For this review, take the finished solid that the model builds, in its own axes (mm). A direction names the side the tool comes from. Give positions to 0.01 mm unless a question says otherwise; leave off trailing zeros. Write each loop counter-clockwise with the first axis right and the second up, starting at its lowest first coordinate (ties: lowest second). Pieces come first, ordered by that corner, then holes. Notation, with made-up numbers: (31.25, 12.25) -> (45.25, 12.25) arc R21 ccw to (45.25, 39.25) -> close; hole circle Ø2 at (13, 46). An arc over 180 degrees is marked (long way). Write item = value, one per line.
```python
from build123d import *

# Parameters (mm, degrees)
SKETCH1_W                    = 320
SKETCH1_H                    = 90.51
CHASSIS_BASE_DEPTH           = 5
SKETCH3_W                    = 2
SKETCH3_H                    = 275
LATERAL_GUARD_DEPTH          = 3
DRIVE_ATTACHMENT_POINT_REACH = 10
SKETCH4_R                    = 3
CUT_EXTRUDE2_REACH           = 7
SKETCH5_R                    = 6.5
SKETCH5_R_2                  = 1
SKETCH6_W                    = 30
SKETCH6_H                    = 30
BOSS_EXTRUDE1_DEPTH          = 90.51
CUT_EXTRUDE3_REACH           = 32
SKETCH7_W                    = 60
SKETCH7_H                    = 30
FILLET3_R                    = 0.5
FILLET4_R                    = 2
SKETCH9_R                    = 0.875
CUT_EXTRUDE5_DEPTH           = 5
SKETCH10_R                   = 0.875
CUT_EXTRUDE6_DEPTH           = 5
SKETCH11_R                   = 0.875
CUT_EXTRUDE7_DEPTH           = 5
SKETCH12_R                   = 0.875
CUT_EXTRUDE8_DEPTH           = 5
SKETCH13_R                   = 0.875
CUT_EXTRUDE9_DEPTH           = 5
SKETCH14_R                   = 0.875
CUT_EXTRUDE10_DEPTH          = 5
BOSS_EXTRUDE2_DEPTH          = 1.6
SKETCH17_R                   = 10.925
CUT_EXTRUDE12_DEPTH          = 91.51
SKETCH18_W                   = 18
SKETCH18_H                   = 15
CUT_EXTRUDE13_DEPTH          = 6.0000001
SKETCH23_R                   = 1.5
CUT_EXTRUDE18_DEPTH          = 35


with BuildPart() as part:
    # Sketch1 → Chassis Base (new body)
    with BuildSketch(Plane(origin=(0, 0, 0), x_dir=(0, 1, 0), z_dir=(0, 0, 1))):
        Rectangle(SKETCH1_W, SKETCH1_H)
    extrude(amount=CHASSIS_BASE_DEPTH)

    # Sketch3 → Lateral Guard (add)
    with BuildSketch(Plane.XY.offset(5)):
        with Locations((-44.255, 7.5)):
            Rectangle(SKETCH3_W, SKETCH3_H)
        with Locations((44.255, 7.5)):
            Rectangle(SKETCH3_W, SKETCH3_H)
    extrude(amount=LATERAL_GUARD_DEPTH)

    # Sketch4 → Drive Attachment Point (cut, up to next)
    with BuildSketch(Plane(origin=(0, 0, 0), x_dir=(1, 0, 0), z_dir=(0, 0, -1)), mode=Mode.PRIVATE) as drive_attachment_point_sk1:
        with Locations((0, -29.7)):
            Circle(SKETCH4_R)
    drive_attachment_point_tool1 = extrude(drive_attachment_point_sk1.sketch, amount=-DRIVE_ATTACHMENT_POINT_REACH, mode=Mode.PRIVATE) & part.part
    add(drive_attachment_point_tool1.solids().sort_by_distance((0, 29.7, 0))[0], mode=Mode.SUBTRACT)
    # Sketch4 → Drive Attachment Point (cut, up to next)
    with BuildSketch(Plane(origin=(0, 0, 0), x_dir=(1, 0, 0), z_dir=(0, 0, -1)), mode=Mode.PRIVATE) as drive_attachment_point_sk2:
        with Locations((-20.08, 30)):
            Circle(SKETCH4_R)
    drive_attachment_point_tool2 = extrude(drive_attachment_point_sk2.sketch, amount=-DRIVE_ATTACHMENT_POINT_REACH, mode=Mode.PRIVATE) & part.part
    add(drive_attachment_point_tool2.solids().sort_by_distance((-20.08, -30, 0))[0], mode=Mode.SUBTRACT)
    # Sketch4 → Drive Attachment Point (cut, up to next)
    with BuildSketch(Plane(origin=(0, 0, 0), x_dir=(1, 0, 0), z_dir=(0, 0, -1)), mode=Mode.PRIVATE) as drive_attachment_point_sk3:
        with Locations((20.08, 30)):
            Circle(SKETCH4_R)
    drive_attachment_point_tool3 = extrude(drive_attachment_point_sk3.sketch, amount=-DRIVE_ATTACHMENT_POINT_REACH, mode=Mode.PRIVATE) & part.part
    add(drive_attachment_point_tool3.solids().sort_by_distance((20.08, -30, 0))[0], mode=Mode.SUBTRACT)
    # Sketch4 → Drive Attachment Point (cut, up to next)
    with BuildSketch(Plane(origin=(0, 0, 0), x_dir=(1, 0, 0), z_dir=(0, 0, -1)), mode=Mode.PRIVATE) as drive_attachment_point_sk4:
        with Locations((0, 49.3)):
            Circle(SKETCH4_R)
    drive_attachment_point_tool4 = extrude(drive_attachment_point_sk4.sketch, amount=-DRIVE_ATTACHMENT_POINT_REACH, mode=Mode.PRIVATE) & part.part
    add(drive_attachment_point_tool4.solids().sort_by_distance((0, -49.3, 0))[0], mode=Mode.SUBTRACT)
    # Sketch4 → Drive Attachment Point (cut, up to next)
    with BuildSketch(Plane(origin=(0, 0, 0), x_dir=(1, 0, 0), z_dir=(0, 0, -1)), mode=Mode.PRIVATE) as drive_attachment_point_sk5:
        with Locations((-20.08, -10.4)):
            Circle(SKETCH4_R)
    drive_attachment_point_tool5 = extrude(drive_attachment_point_sk5.sketch, amount=-DRIVE_ATTACHMENT_POINT_REACH, mode=Mode.PRIVATE) & part.part
    add(drive_attachment_point_tool5.solids().sort_by_distance((-20.08, 10.4, 0))[0], mode=Mode.SUBTRACT)
    # Sketch4 → Drive Attachment Point (cut, up to next)
    with BuildSketch(Plane(origin=(0, 0, 0), x_dir=(1, 0, 0), z_dir=(0, 0, -1)), mode=Mode.PRIVATE) as drive_attachment_point_sk6:
        with Locations((20.08, -10.4)):
            Circle(SKETCH4_R)
    drive_attachment_point_tool6 = extrude(drive_attachment_point_sk6.sketch, amount=-DRIVE_ATTACHMENT_POINT_REACH, mode=Mode.PRIVATE) & part.part
    add(drive_attachment_point_tool6.solids().sort_by_distance((20.08, 10.4, 0))[0], mode=Mode.SUBTRACT)

    # Sketch5 → Cut-Extrude2 (cut, up to next)
    with BuildSketch(Plane.XY.offset(5), mode=Mode.PRIVATE) as cut_extrude2_sk1:
        with Locations((0, 148)):
            Circle(SKETCH5_R)
    cut_extrude2_tool1 = extrude(cut_extrude2_sk1.sketch, amount=-CUT_EXTRUDE2_REACH, mode=Mode.PRIVATE) & part.part
    add(cut_extrude2_tool1.solids().sort_by_distance((0, 148, 5))[0], mode=Mode.SUBTRACT)
    # Sketch5 → Cut-Extrude2 (cut, up to next)
    with BuildSketch(Plane.XY.offset(5), mode=Mode.PRIVATE) as cut_extrude2_sk2:
        with Locations((-17.5, 140.5)):
            Circle(SKETCH5_R_2)
    cut_extrude2_tool2 = extrude(cut_extrude2_sk2.sketch, amount=-CUT_EXTRUDE2_REACH, mode=Mode.PRIVATE) & part.part
    add(cut_extrude2_tool2.solids().sort_by_distance((-17.5, 140.5, 5))[0], mode=Mode.SUBTRACT)
    # Sketch5 → Cut-Extrude2 (cut, up to next)
    with BuildSketch(Plane.XY.offset(5), mode=Mode.PRIVATE) as cut_extrude2_sk3:
        with Locations((17.5, 140.5)):
            Circle(SKETCH5_R_2)
    cut_extrude2_tool3 = extrude(cut_extrude2_sk3.sketch, amount=-CUT_EXTRUDE2_REACH, mode=Mode.PRIVATE) & part.part
    add(cut_extrude2_tool3.solids().sort_by_distance((17.5, 140.5, 5))[0], mode=Mode.SUBTRACT)

    # Sketch6 → Boss-Extrude1 (add)
    with BuildSketch(Plane.YZ.offset(45.255)):
        with Locations((-145, 15)):
            Rectangle(SKETCH6_W, SKETCH6_H)
    extrude(amount=-BOSS_EXTRUDE1_DEPTH)

    # Sketch7 → Cut-Extrude3 (cut, up to next)
    with BuildSketch(Plane.XY.offset(30), mode=Mode.PRIVATE) as cut_extrude3_sk1:
        with Locations((0, -145)):
            Rectangle(SKETCH7_W, SKETCH7_H)
    cut_extrude3_tool1 = extrude(cut_extrude3_sk1.sketch, amount=-CUT_EXTRUDE3_REACH, mode=Mode.PRIVATE) & part.part
    add(cut_extrude3_tool1.solids().sort_by_distance((0, -145, 30))[0], mode=Mode.SUBTRACT)

    # Fillet3
    fillet3_edges = [part.edges().sort_by_distance(p)[0] for p in [
        (-45.255, 7.5, 8),
        (-43.255, 7.5, 8),
        (45.255, 7.5, 8),
        (43.255, 7.5, 8),
    ]]
    fillet(fillet3_edges, radius=FILLET3_R)

    # Fillet4
    fillet4_edges = [part.edges().sort_by_distance(p)[0] for p in [
        (37.6275, -130, 30),
        (-37.6275, -130, 30),
    ]]
    fillet(fillet4_edges, radius=FILLET4_R)

    # Sketch9 → Cut-Extrude5 (cut)
    with BuildSketch(Plane.XY.offset(30)):
        with Locations((-37.6275, -146)):
            Circle(SKETCH9_R)
    extrude(amount=-CUT_EXTRUDE5_DEPTH, mode=Mode.SUBTRACT)

    # Sketch10 → Cut-Extrude6 (cut)
    with BuildSketch(Plane.XZ.offset(160)):
        with Locations((-37.6275, 15)):
            Circle(SKETCH10_R)
    extrude(amount=-CUT_EXTRUDE6_DEPTH, mode=Mode.SUBTRACT)

    # Sketch11 → Cut-Extrude7 (cut)
    with BuildSketch(Plane(origin=(0, 0, 0), x_dir=(1, 0, 0), z_dir=(0, 0, -1))):
        with Locations((-37.6275, 148.599605515)):
            Circle(SKETCH11_R)
    extrude(amount=-CUT_EXTRUDE7_DEPTH, mode=Mode.SUBTRACT)

    # Sketch12 → Cut-Extrude8 (cut)
    with BuildSketch(Plane(origin=(0, 0, 0), x_dir=(1, 0, 0), z_dir=(0, 0, -1))):
        with Locations((37.6275, 145)):
            Circle(SKETCH12_R)
    extrude(amount=-CUT_EXTRUDE8_DEPTH, mode=Mode.SUBTRACT)

    # Sketch13 → Cut-Extrude9 (cut)
    with BuildSketch(Plane.XZ.offset(160)):
        with Locations((37.6275, 15)):
            Circle(SKETCH13_R)
    extrude(amount=-CUT_EXTRUDE9_DEPTH, mode=Mode.SUBTRACT)

    # Sketch14 → Cut-Extrude10 (cut)
    with BuildSketch(Plane.XY.offset(30)):
        with Locations((37.6275, -146)):
            Circle(SKETCH14_R)
    extrude(amount=-CUT_EXTRUDE10_DEPTH, mode=Mode.SUBTRACT)

    # Sketch15 → Boss-Extrude2 (add)
    with BuildSketch(Plane.XY.offset(5)):
        with BuildLine():
            Line((-17.021586315, 136.436061109), (17.021586315, 136.436061109))
            ThreePointArc((17.021586315, 136.436061109), (0, 123), (-17.021586315, 136.436061109))
        make_face()
    extrude(amount=BOSS_EXTRUDE2_DEPTH)

    # Sketch17 → Cut-Extrude12 (cut, through all)
    with BuildSketch(Plane(origin=(-45.255, 0, 0), x_dir=(0, -1, 0), z_dir=(-1, 0, 0))):
        with Locations((145, 15)):
            Circle(SKETCH17_R)
    extrude(amount=-CUT_EXTRUDE12_DEPTH, mode=Mode.SUBTRACT)

    # Sketch18 → Cut-Extrude13 (cut, through all)
    with BuildSketch(Plane.XY.offset(5)):
        with Locations((21, -122.5)):
            Rectangle(SKETCH18_W, SKETCH18_H)
        with Locations((-21, -122.5)):
            Rectangle(SKETCH18_W, SKETCH18_H)
    extrude(amount=-CUT_EXTRUDE13_DEPTH, mode=Mode.SUBTRACT)

    # Sketch21 → Revolve1 (revolve)
    with BuildSketch(Plane.YZ):
        with BuildLine():
            Line((-118, 40), (-118, 5))
            Line((-118, 5), (-106.234133627, 4.682586024))
            add(Edge.make_bspline(
                [(-115, 40), (-114.798550354, 20.795762888), (-106.234133627, 4.682586024)],
                knots=[0, 0, 0, 1, 1, 1], degree=2))
            Line((-115, 40), (-118, 40))
        make_face()
    revolve(axis=Axis((0, -118, 40), (0, 0, -1)))

    # Sketch23 → Cut-Extrude18 (cut)
    with BuildSketch(Plane(origin=(0, 0, 40), x_dir=(0, 1, 0), z_dir=(0, 0, 1))):
        with Locations((-118, 0)):
            Circle(SKETCH23_R)
    extrude(amount=-CUT_EXTRUDE18_DEPTH, mode=Mode.SUBTRACT)


solid = part.part
```
(1) Tool access review of faces 1 (the face through (30, -138, 5)), 2 (the face through (17.083, -30.132, 2.465)), 3 (the face through (0, 123, 6)): name each direction out of +Z, -Z, +X, -X, +Y, -Y from which nothing blocks a thin tool from reaching the whole face with its end or side.
Answers below:
face_1 = +Z, -Z, -Y
face_2 = +Z, -Z
face_3 = +Z
(2) To check wall thickness, follow probe 1 along Y at (x, z) = (-20.08, 1.95); probe 2 along Y at (x, z) = (0, 3.3); probe 3 along X at (y, z) = (-158.1, 15) (1 decimal). State the ranges of each line that lie inside material, in increasing order.
Answers below:
probe_1 = -115 to -33, -27 to 7.4, 13.4 to 160
probe_2 = -130 to -52.3, -46.3 to 26.7, 32.7 to 141.5, 154.5 to 160
probe_3 = -45.3 to -38.5, -36.8 to -30, 30 to 36.8, 38.5 to 45.3
(3) Take a section at A-A (y = -49.3). Write out the cut boundary in (x, z) (3 decimals).
Answers below:
outline = (-45.255, 0) -> (-3, 0) -> (-3, 5) -> (-43.255, 5) -> (-43.255, 7.5) arc R0.5 ccw to (-43.755, 8) -> (-44.755, 8) arc R0.5 ccw to (-45.255, 7.5) -> close; (3, 0) -> (45.255, 0) -> (45.255, 7.5) arc R0.5 ccw to (44.755, 8) -> (43.755, 8) arc R0.5 ccw to (43.255, 7.5) -> (43.255, 5) -> (3, 5) -> close
(4) For pin 1 (10 mm diameter, centred on x = 6, z = 7.5, fed in from -Y); pin 2 (4 mm diameter, centred on x = -3.5, y = 129, fed in from +Z); pin 3 (1 mm diameter, centred on x = 44, z = 6, fed in from +Y), all flat-tipped, find the tip position at first contact; note any pin that passes through.
Answers below:
pin_1 = -130
pin_2 = 6.6
pin_3 = 145
(5) The part is to be moulded in two halves that separate along X. For faces 4 (the face through (-45.255, -24, 6)), 5 (the face through (-30, -138, 5)), 6 (the face through (45.255, -24, 6)), 7 (the face through (36, -160, 15)), say which applies: released by +X, released by -X, zero draft, split by the parting line, or undercut.
Answers below:
face_4 = released by -X
face_5 = undercut
face_6 = released by +X
face_7 = zero draft
(6) Take a section at C-C (z = 19). Count the separate pieces of the cut face and the enclosed holes in it, plus the area to 3 significant figures.
Answers below:
separate_pieces = 5
enclosed_holes = 1
area = 400 mm^2
(7) Take a section at B-B (y = 24). Write out the cut boundary in (x, z) (3 decimals), plus the area to 3 significant figures.
Answers below:
outline = (-45.255, 0) -> (45.255, 0) -> (45.255, 7.5) arc R0.5 ccw to (44.755, 8) -> (43.755, 8) arc R0.5 ccw to (43.255, 7.5) -> (43.255, 5) -> (-43.255, 5) -> (-43.255, 7.5) arc R0.5 ccw to (-43.755, 8) -> (-44.755, 8) arc R0.5 ccw to (-45.255, 7.5) -> close
area = 464 mm^2
